Answer from the drawing. Dimensions are ordinates in mm from the lowest x, y and z of the part. A direction names the side the tool comes from. Coordinates: 2 decimals unless noted, no trailing zeros. Order: outer loops, then holes, each group sorted by start corner. A loop starts at its lowest first (then second) coordinate and runs counter-clockwise, first axis right, second up. Notation, with made-up numbers: (4, -38) - (17, -38) arc R14 cw to (17, -19) - close; hole circle Ø6 at (83.25, -38). An arc over 180 degrees is marked (long way). Use a Markdown table: item, result. Add a question column.
Item 1: The part is cut by section D-D, the plane y = 9.25. State how many separate pieces and enclosed holes the cut face has, then the cut area to 3 significant figures.
Item 2: The part is cut by section C-C, the plane y = 12.5. Give the vertices of the cut face in (x, z) (1 decimal), then the cut area to 3 significant figures.
Item 3: Find the intervals of material crossed by line 1 along Z through (x, y) = (30, 1.25); line 2 along Z through (x, y) = (14.5, 7) (1 decimal); line 3 along Z through (x, y) = (15, 7) (1 decimal), in increasing order.
Item 4: The part is cut by section B-B, the plane z = 30. Give the vertices of the cut face in (x, y) (1 decimal), then the cut area to 3 significant figures.
Item 5: For the marked faces 1 and 2, determine the directions among +Z, -Z, +X, -X, +Y, -Y from which every point of the face is accessible in a straight line to the end or side of a thin tool.
Item 6: The part is cut by section A-A, the plane x = 30. Give the vertices of the cut face in (y, z) (1 decimal).
Item 7: Flat-ended cylindrical pins translate along their axes: P1, Ø4, axis at x = 53, y = 9.5, coming from the +Z side (1 decimal); P2, Ø3.5, axis at x = 44.89, z = 9.5, coming from the +Y side; P3, Ø4, axis at x = 30, z = 30, coming from the -Y side; P4, Ø1.5, axis at x = 49.5, y = 5.5, coming from the +Z side. Find the tip coordinate at first contact, or state that the pin passes through.
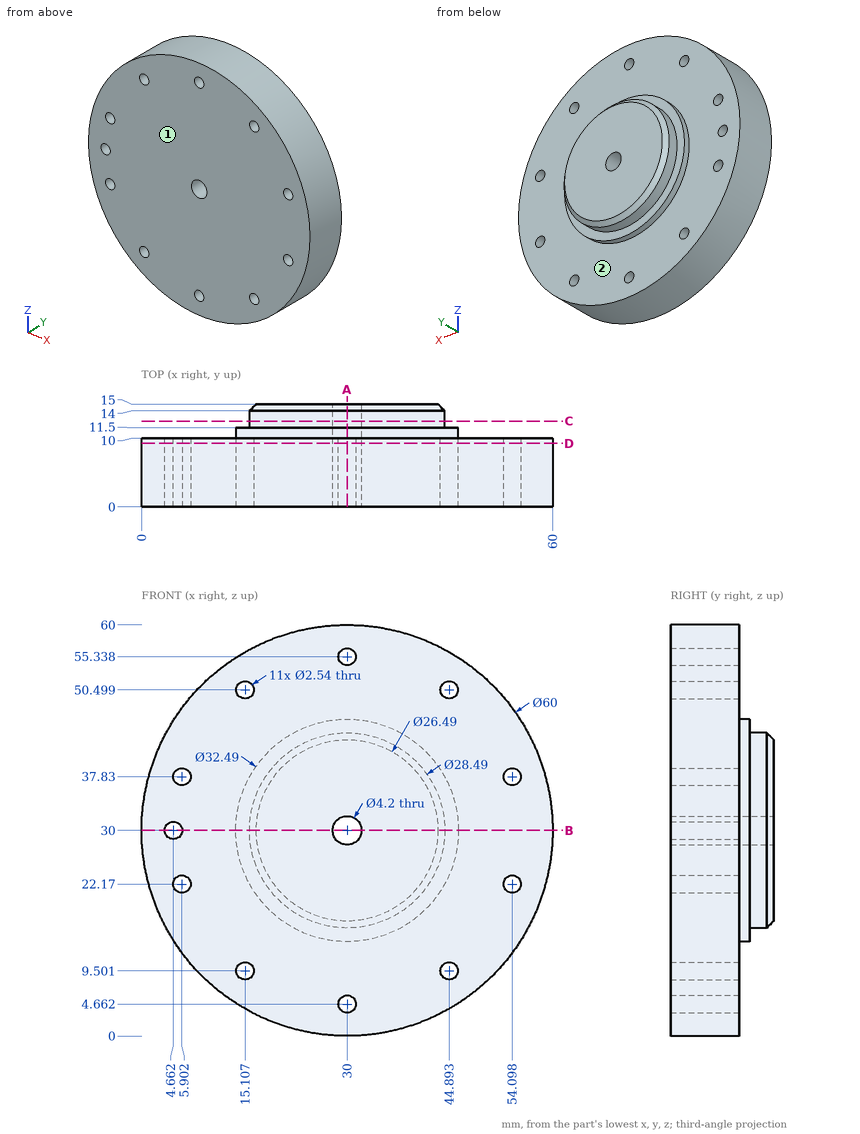
Solution:
| question | item | result |
|---|---|---|
| 1 | separate pieces | 1 |
| 1 | enclosed holes | 12 |
| 1 | area | 2,760 mm2 |
| 2 | outline | circle Ø28.5 at (30, 30); hole circle Ø4.2 at (30, 30) |
| 2 | area | 624 mm2 |
| 3 | line 1 | z = 0 to 3.39, 5.93 to 27.9, 32.1 to 54.07, 56.61 to 60 |
| 3 | line 2 | z = 4.3 to 8.4, 10.6 to 49.4, 51.6 to 55.7 |
| 3 | line 3 | z = 4 to 8.2, 10.8 to 49.2, 51.8 to 56 |
| 4 | outline | (0, 0) - (3.4, 0) - (3.4, 10) - (0, 10) - close; (5.9, 0) - (27.9, 0) - (27.9, 15) - (16.8, 15) - (15.8, 14) - (15.8, 11.5) - (13.8, 11.5) - (13.8, 10) - (5.9, 10) - close; (32.1, 0) - (60, 0) - (60, 10) - (46.2, 10) - (46.2, 11.5) - (44.2, 11.5) - (44.2, 14) - (43.2, 15) - (32.1, 15) - close |
| 4 | area | 659 mm2 |
| 5 | face 1 | +Z, -Z, +X, -X, -Y |
| 5 | face 2 | +Y |
| 6 | outline | (0, 0) - (10, 0) - (10, 3.4) - (0, 3.4) - close; (0, 5.9) - (10, 5.9) - (10, 13.8) - (11.5, 13.8) - (11.5, 15.8) - (14, 15.8) - (15, 16.8) - (15, 27.9) - (0, 27.9) - close; (0, 32.1) - (15, 32.1) - (15, 43.2) - (14, 44.2) - (11.5, 44.2) - (11.5, 46.2) - (10, 46.2) - (10, 54.1) - (0, 54.1) - close; (0, 56.6) - (10, 56.6) - (10, 60) - (0, 60) - close |
| 7 | P1 | stops at z = 51.4 |
| 7 | P2 | stops at y = 10 |
| 7 | P3 | passes through |
| 7 | P4 | stops at z = 53.42 |
